Input: part model. Units: mm. Frame: model coordinates. A direction names the side the tool comes from. Give positions to 0.01 mm unless a question says otherwise; leave off trailing zeros. Order: outer loops, then holes, each group sorted by start corner. A loop starts at its lowest first (then second) coordinate and runs counter-clockwise, first axis right, second up. Notation, with made-up numbers: (-23, 77.25) - (15, 77.25) arc R30 cw to (15, 110.25) - close; hole circle Ø4 at (-34.5, 10.25). An arc over 180 degrees is marked (long way). Use a Markdown table: item, result.
from build123d import *

# Parameters (mm, degrees)
BOSS_EXTRUDE1_DEPTH = 3
FILLET1_R           = 0.5
SKETCH2_R           = 2
CUT_EXTRUDE1_DEPTH  = 10
SKETCH3_R           = 2
CUT_EXTRUDE2_DEPTH  = 3
CUT_EXTRUDE3_START  = 50
SKETCH4_R           = 1.54375
CUT_EXTRUDE3_DEPTH  = 30
CUT_EXTRUDE4_START  = -1.5
CUT_EXTRUDE4_DEPTH  = 0.5


with BuildPart() as part:
    # Sketch1 → Boss-Extrude1 (new body)
    with BuildSketch(Plane.XY):
        with BuildLine():
            Line((-3.966766701, 3.043807145), (-1.983383351, 1.521903573))
            ThreePointArc((-1.983383351, 1.521903573), (2.5, 0), (-1.983383351, -1.521903573))
            Line((-1.983383351, -1.521903573), (-3.966766701, -3.043807145))
            ThreePointArc((-3.966766701, -3.043807145), (-2.211443451, -4.484363708), (0, -5))
            Line((0, -5), (20, -5))
            ThreePointArc((20, -5), (25, 0), (20, 5))
            Line((20, 5), (0, 5))
            ThreePointArc((0, 5), (-2.211443451, 4.484363708), (-3.966766701, 3.043807145))
        make_face()
    extrude(amount=BOSS_EXTRUDE1_DEPTH)

    # Fillet1
    fillet1_edges = [part.edges().sort_by_distance(p)[0] for p in [
        (-1.983383351, -1.521903573, 1.5),
        (-1.983383351, 1.521903573, 1.5),
    ]]
    fillet(fillet1_edges, radius=FILLET1_R)

    # Sketch2 → Cut-Extrude1 (cut)
    with BuildSketch(Plane.XY.offset(3)):
        with Locations((20, 0)):
            Circle(SKETCH2_R)
    extrude(amount=-CUT_EXTRUDE1_DEPTH, mode=Mode.SUBTRACT)

    # Sketch3 → Cut-Extrude2 (cut)
    with BuildSketch(Plane.XY.offset(3)):
        with Locations((12, 0)):
            Circle(SKETCH3_R)
    extrude(amount=-CUT_EXTRUDE2_DEPTH, mode=Mode.SUBTRACT)

    # Sketch4 → Cut-Extrude3 (cut)
    with BuildSketch(Plane(origin=(0, 0, 0), x_dir=(0, 0, -1), z_dir=(1, 0, 0)).offset(CUT_EXTRUDE3_START)):
        with Locations((-1.5, 0)):
            Circle(SKETCH4_R)
    extrude(amount=-CUT_EXTRUDE3_DEPTH, mode=Mode.SUBTRACT)

    # Sketch5 → Cut-Extrude4 (cut, symmetric)
    with BuildSketch(Plane(origin=(0, 0, 0), x_dir=(-1, 0, 0), z_dir=(0, 0, -1)).offset(CUT_EXTRUDE4_START)):
        with BuildLine():
            Line((-21.608635668, -3.66227952), (-23.404072372, -3.66227952))
            ThreePointArc((-23.404072372, -3.66227952), (-21.828743065, -4.653568394), (-20, -5))
            Line((-20, -5), (0, -5))
            Line((0, -5), (3, -5))
            Line((3, -5), (3, -4))
            Line((3, -4), (-20, -4))
            ThreePointArc((-20, -4), (-20.821852152, -3.914659505), (-21.608635668, -3.66227952))
        make_face()
    extrude(amount=CUT_EXTRUDE4_DEPTH, both=True, mode=Mode.SUBTRACT)


solid = part.part
1. Section query A-A (y = 0). Return loops of the section in (x, z).
Response:
| item | result |
|---|---|
| outline | (2.5, 0) - (10, 0) - (10, 3) - (2.5, 3) - close; (14, 0) - (18, 0) - (18, 3) - (14, 3) - close |
2. Mould query, pull axis Y, two halves, no side actions, for faces 5 (the face through (8.3, -4, 1.5)), 6 (the face through (10, 5, 1)), 7 (the face through (2.5, 0.1, 1.5)), 8 (the face through (-3.145, -2.414, 1.479)). Classes: pulls with the +Y half, pulls with the -Y half, needs draft (parallel to the pull), parting line crosses it, or undercut.
Response:
| item | result |
|---|---|
| face 5 | pulls with the -Y half |
| face 6 | pulls with the +Y half |
| face 7 | undercut |
| face 8 | undercut |
3. Material intervals for line 1 along Y through (x, z) = (0, 0.95); line 2 along X through (y, z) = (1.75, 1.3); line 3 along Y through (x, z) = (20, 1.6), sorted ascending.
Response:
| item | result |
|---|---|
| line 1 | y = -5 to -2.5, 2.5 to 5 |
| line 2 | x = -2.27 to -1.82, 1.79 to 11.03, 12.97 to 19.03, 20.97 to 24.68 |
| line 3 | y = -4 to -2, 2 to 5 |
4. Section query C-C (z = 2.4). Return loops of the section in (x, y), then the cut area to 3 significant figures.
Response:
| item | result |
|---|---|
| outline | (-3.97, -3.04) arc R5 ccw to (0, -5) - (20, -5) arc R5 ccw to (24.84, -1.25) - (21.56, -1.25) arc R2 cw (long way) to (21.56, 1.25) - (24.84, 1.25) arc R5 ccw to (20, 5) - (0, 5) arc R5 ccw to (-3.97, 3.04) - (-2.35, 1.8) arc R0.5 ccw to (-1.7, 1.83) arc R2.5 cw (long way) to (-1.7, -1.83) arc R0.5 ccw to (-2.35, -1.8) - close; hole circle Ø4 at (12, 0) |
| area | 214 mm^2 |
5. Set-up query: faces 1 (the face through (23.155, -1.543, 1.529)), 2 (the face through (10, 1, 3)), 3 (the face through (20.811, -3.917, 1.493)), 4 (the face through (-3.17, 2.43, 1.48)). Return all of +Z, -Z, +X, -X, +Y, -Y with unobstructed straight access to the full face (end or side cutting, diameter ignored); none if empty.
Response:
| item | result |
|---|---|
| face 1 | +X |
| face 2 | +Z, +X, -X, +Y, -Y |
| face 3 | +X, -Y |
| face 4 | +Z, -Z, -X |
6. Section query B-B (x = 16.5). Return loops of the section in (y, z), then the cut area to 3 significant figures.
Response:
| item | result |
|---|---|
| outline | (-5, 0) - (5, 0) - (5, 3) - (-5, 3) - (-5, 2) - (-4, 2) - (-4, 1) - (-5, 1) - close |
| area | 29.0 mm^2 |
7. Section query D-D (x = 12). Return loops of the section in (y, z).
Response:
| item | result |
|---|---|
| outline | (-5, 0) - (-2, 0) - (-2, 3) - (-5, 3) - (-5, 2) - (-4, 2) - (-4, 1) - (-5, 1) - close; (2, 0) - (5, 0) - (5, 3) - (2, 3) - close |
8. Pin query (flat end, axial travel): pin 1 (1 mm diameter, centred on y = 1.5, z = 0.5, fed in from -X); pin 2 (0.5 mm diameter, centred on x = 6.5, z = 1.5, fed in from -Y). Return the tip coordinate at first contact, or that it passes through.
Response:
| item | result |
|---|---|
| pin 1 | stops at x = -2.61 |
| pin 2 | stops at y = -4 |
